from build123d import *

# Parameters (mm, degrees)
SKETCH_1_R          = 3.25
EXTRUDE_1_DEPTH     = 13
SKETCH_2_R          = 5.375758968
EXTRUDE_2_DEPTH     = 5
EXTRUDE_2_DRAFT     = -23
SKETCH_3_R          = 1.7
CUT_EXTRUDE_1_DEPTH = 16.059799765
FILLET_1_R          = 1
FILLET_2_R          = 0.5
FILLET_3_R          = 1


with BuildPart() as part:
    # 草图1 → 凸台-拉伸1 (new body)
    with BuildSketch(Plane.XY):
        with Locations(Location((0, 0, 0), (0, 0, 180))):
            Circle(SKETCH_1_R)
    extrude(amount=EXTRUDE_1_DEPTH)


with BuildPart() as extrude_2_tool:
    # 草图2 → 凸台-拉伸2 (with draft: the straight prism first)
    with BuildSketch(Plane(origin=(0, 0, 0), x_dir=(-1, 0, 0), z_dir=(0, 0, -1))):
        Circle(SKETCH_2_R)
    extrude(amount=-EXTRUDE_2_DEPTH)
    # 凸台-拉伸2: the draft: its side faces are tilted about the plane it starts from
    extrude_2_sides = [extrude_2_tool.faces().sort_by_distance(p)[0] for p in [
        (5.375758968, 0, 2.5),
    ]]
    draft(extrude_2_sides, Plane(origin=(0, 0, 0), x_dir=(-1, 0, 0), z_dir=(0, 0, -1)), EXTRUDE_2_DRAFT)


with BuildPart() as part_1:
    add(part.part)

    # 凸台-拉伸2: add extrude_2_tool
    add(extrude_2_tool.part)

    # 草图3 → 切除-拉伸1 (cut, through all)
    with BuildSketch(Plane(origin=(0, 0, 0), x_dir=(-1, 0, 0), z_dir=(0, 0, -1))):
        Circle(SKETCH_3_R)
    extrude(amount=-CUT_EXTRUDE_1_DEPTH, mode=Mode.SUBTRACT)

    # 圆角1
    fillet_1_edges = [part_1.edges().sort_by_distance(p)[0] for p in [
        (3.25, 0, 13),
    ]]
    fillet(fillet_1_edges, radius=FILLET_1_R)

    # 圆角2
    fillet_2_edges = [part_1.edges().sort_by_distance(p)[0] for p in [
        (5.375758968, 0, 0),
    ]]
    fillet(fillet_2_edges, radius=FILLET_2_R)

    # 圆角3
    # the kernel refuses this fillet: 1 mm, written as the material it takes off along each edge
    with BuildSketch(Plane(origin=(0, 0, 5), x_dir=(-1, 0, 0), z_dir=(0, -1, 0))) as fillet_3_piece_1:
        with BuildLine():
            CenterArc((2.363183754, 0.46212222), FILLET_3_R, 332.475864529, 4.524135471)
            Line((3.25, 0), (3.253384887, 0))
            Line((3.253384887, 0), (3.283688608, 0.071391091))
        make_face()
    revolve(axis=Axis((0, 0, 5), (0, 0, -1)), mode=Mode.SUBTRACT)


solid = part_1.part
Read the model definition and answer for the solid it produces. Units are mm, in the model's axes. Coordinates: 2 decimals unless noted, no trailing zeros. Write each loop counter-clockwise with the first axis right and the second up, starting at its lowest first coordinate (ties: lowest second). Pieces come first, ordered by that corner, then holes. Notation, with made-up numbers: M 3,55.5 L 58,55.5 A21 ccw 58,64.5 Z; hole C -24.5,0.25 d11. An arc over 180 degrees is marked long. Use a Markdown table: item, result.
Q1. Each of these flat-tipped pins is pushed along its axis until it touches: pin 1 Ø3 at (y, z) = (-2, 8.5) entering from -X; pin 2 Ø5 at (y, z) = (1, 4) entering from +X; pin 3 Ø2 at (y, z) = (-3.5, 6.5) entering from -X. Where does it stop, or does it pass through?
Answer block:
| item | result |
|---|---|
| pin 1 | stops at x = -3.21 |
| pin 2 | stops at x = 4.69 |
| pin 3 | stops at x = -2.08 |
Q2. Straight lines are drawn through the part: L1, parallel to Y at x = 0, z = 10.25; L2, parallel to Y at x = 0, z = 4.25; L3, parallel to X at y = -0.25, z = 3.5. For each, find the intervals that lie inside material, in ascending order. Write a range as [from, to].
Answer block:
| item | result |
|---|---|
| L1 | y = [-3.25, -1.7], [1.7, 3.25] |
| L2 | y = [-3.57, -1.7], [1.7, 3.57] |
| L3 | x = [-3.88, -1.68], [1.68, 3.88] |
Q3. The part is cut by section D-D, the plane z = 4.75. Write down the section's boundary in (x, y).
Answer block:
| item | result |
|---|---|
| outline | C 0,0 d6.72; hole C 0,0 d3.4 |
Q4. The part is cut by section C-C, the plane z = 7. Write down the section's boundary in (x, y), then the cut area to 3 significant figures.
Answer block:
| item | result |
|---|---|
| outline | C 0,0 d6.5; hole C 0,0 d3.4 |
| area | 24.1 mm2 |
Q5. Determine the mould class of faces 1 (the face through (2.579, 1.978, 8.451)), 2 (the face through (-2, 0, 0)), 3 (the face through (0.37, -1.66, 6.41)) for opening direction Y: released by +Y, released by -Y, zero draft, split by the parting line, or undercut.
Answer block:
| item | result |
|---|---|
| face 1 | split by the parting line |
| face 2 | zero draft |
| face 3 | undercut |
Q6. The part is cut by section A-A, the plane y = 0. Write down the section's boundary in (x, z).
Answer block:
| item | result |
|---|---|
| outline | M -5.08,0.7 A0.5 ccw -4.62,0 L -1.7,0 L -1.7,13 L -2.25,13 A1 ccw -3.25,12 L -3.25,5 A1 ccw -3.28,4.93 Z; M 1.7,0 L 4.62,0 A0.5 ccw 5.08,0.7 L 3.28,4.93 A1 ccw 3.25,5 L 3.25,12 A1 ccw 2.25,13 L 1.7,13 Z |
